```python
from build123d import *

# Parameters (mm, degrees)
F0_R     = 18.5
F1_DEPTH = 8
F2_R     = 30
F3_R     = 2.5
F4_R     = 20
F5_R     = 2
F6_SIZE2 = 0.0727940469
F6_SIZE  = 0.2


with BuildPart() as f1:
    # F0 (on Top) → F1 (new body)
    with BuildSketch(Plane.XY):
        with BuildLine():
            Line((0, 105), (0, 0))
            Line((0, 0), (75, 0))
            Line((75, 0), (75, 105))
            Line((75, 105), (62.5, 105))
            ThreePointArc((62.5, 105), (37.5, 80), (12.5, 105))
            Line((12.5, 105), (0, 105))
        make_face()
        with Locations((37.5, 30)):
            Circle(F0_R, mode=Mode.SUBTRACT)
        with BuildLine():
            Line((0, 140), (0, 105))
            Line((0, 105), (12.5, 105))
            ThreePointArc((12.5, 105), (37.5, 130), (62.5, 105))
            Line((62.5, 105), (75, 105))
            Line((75, 105), (75, 140))
            Line((75, 140), (0, 140))
        make_face()
    extrude(amount=F1_DEPTH)

    # F2
    f2_edges = [f1.edges().sort_by_distance(p)[0] for p in [
        (75, 0, 4),
        (0, 0, 4),
    ]]
    fillet(f2_edges, radius=F2_R)

    # F3
    f3_edges = [f1.edges().sort_by_distance(p)[0] for p in [
        (62.5, 105, 8),
        (19, 30, 8),
    ]]
    fillet(f3_edges, radius=F3_R)

    # F4
    f4_edges = [f1.edges().sort_by_distance(p)[0] for p in [
        (0, 140, 4),
        (75, 140, 4),
    ]]
    fillet(f4_edges, radius=F4_R)

    # F5
    f5_edges = [f1.edges().sort_by_distance(p)[0] for p in [
        (69.142136, 134.142136, 8),
        (37.5, 140, 8),
        (5.857864, 134.142136, 8),
        (0, 75, 8),
        (75, 75, 8),
        (66.213203, 8.786797, 8),
        (37.5, 0, 8),
        (8.786797, 8.786797, 8),
    ]]
    fillet(f5_edges, radius=F5_R)

    # F6
    f6_edges = [f1.edges().sort_by_distance(p)[0] for p in [
        (0, 75, 0),
        (5.857864, 134.142136, 0),
        (8.786797, 8.786797, 0),
        (37.5, 140, 0),
        (37.5, 0, 0),
        (69.142136, 134.142136, 0),
        (66.213203, 8.786797, 0),
        (75, 75, 0),
        (62.5, 105, 0),
        (19, 30, 0),
    ]]
    f6_side = f1.faces().sort_by_distance((37.5, 68.187347, 0))[0]
    chamfer(f6_edges, length=F6_SIZE, length2=F6_SIZE2, reference=f6_side)


solid = f1.part
```
Work out the finished part from the listing and answer in its coordinate system (mm). Give positions to 0.01 mm unless a question says otherwise; leave off trailing zeros. Write each loop counter-clockwise with the first axis right and the second up, starting at its lowest first coordinate (ties: lowest second). Pieces come first, ordered by that corner, then holes. Notation, with made-up numbers: (-14.75, 85) -> (-5.75, 85) arc R23 cw to (-5.75, 107) -> close; hole circle Ø10 at (-10, 41). An arc over 180 degrees is marked (long way). Write each question's results on one line, items separated by ' | '.
1. Each of these flat-tipped pins is pushed along its axis until it touches: pin 1 Ø1.5 at (x, z) = (46.5, 6) entering from -Y; pin 2 Ø1.5 at (x, y) = (23, 126) entering from +Z; pin 3 Ø1 at (x, z) = (67, 1) entering from +Y. Where does it stop, or does it pass through?
Data:
pin 1: y = 0.01 | pin 2: z = 7.68 | pin 3: y = 136.36
2. Find section C-C on y = 105. Determine the outline of the cut face in (x, z).
Data:
outline: (0, 0.07) -> (0.2, 0) -> (12.3, 0) -> (12.5, 0.07) -> (12.5, 5.5) arc R2.5 ccw to (10, 8) -> (2, 8) arc R2 ccw to (0, 6) -> close; (62.5, 0.07) -> (62.7, 0) -> (74.8, 0) -> (75, 0.07) -> (75, 6) arc R2 ccw to (73, 8) -> (65, 8) arc R2.5 ccw to (62.5, 5.5) -> close
3. Find section A-A on x = 37.5. Determine the outline of the cut face in (y, z), and give its area (3 significant figures).
Data:
outline: (0, 0.07) -> (0.2, 0) -> (11.3, 0) -> (11.5, 0.07) -> (11.5, 5.5) arc R2.5 ccw to (9, 8) -> (2, 8) arc R2 ccw to (0, 6) -> close; (48.5, 0.07) -> (48.7, 0) -> (79.8, 0) -> (80, 0.07) -> (80, 5.5) arc R2.5 ccw to (77.5, 8) -> (51, 8) arc R2.5 ccw to (48.5, 5.5) -> close; (130, 0.07) -> (130.2, 0) -> (139.8, 0) -> (140, 0.07) -> (140, 6) arc R2 ccw to (138, 8) -> (132.5, 8) arc R2.5 ccw to (130, 5.5) -> close | area: 417 mm^2
4. Find section B-B on z = 1.75. Determine the outline of the cut face in (x, y).
Data:
outline: (0, 30) arc R30 ccw to (30, 0) -> (45, 0) arc R30 ccw to (75, 30) -> (75, 120) arc R20 ccw to (55, 140) -> (20, 140) arc R20 ccw to (0, 120) -> close; hole circle Ø50 at (37.5, 105); hole circle Ø37 at (37.5, 30)
5. Determine the mould class of faces 1 (the cylindrical face through (54.589, 22.914, 2.748)), 2 (the flat face through (37, 71, 8)), 3 (the flat face through (37, 0, 3)) for opening direction Y: +Y half, -Y half, draft (parallel to the pull), parting line (faces both ways), or undercut.
Data:
face 1: undercut | face 2: draft | face 3: -Y half
6. Straight lines are drawn through the part: L1, parallel to Y at x = 37.5, z = 1.5; L2, parallel to Y at x = 28.5, z = 1.5; L3, parallel to X at y = 29.5, z = 2.25. For each, find the intervals that lie inside material, in ascending order.
Data:
L1: 0 to 11.5, 48.5 to 80, 130 to 140 | L2: 0.04 to 13.84, 46.16 to 81.68, 128.32 to 140 | L3: 0 to 19.01, 55.99 to 75
